from build123d import *

# Parameters (mm, degrees)
SKETCH_W      = 234
SKETCH_H      = 135
PAD_DEPTH     = 5
FILLET_R      = 3
FILLET001_R   = 3
FILLET002_R   = 3
FILLET003_R   = 3
SKETCH001_R   = 3
SKETCH001_R_2 = 5
POCKET_DEPTH  = 5.001


with BuildPart() as part:
    # Sketch → Pad (new body)
    with BuildSketch(Plane.XZ):
        Rectangle(SKETCH_W, SKETCH_H)
    extrude(amount=PAD_DEPTH)

    # Fillet
    fillet_edges = [part.edges().sort_by_distance(p)[0] for p in [
        (117, -2.5, 67.5),
    ]]
    fillet(fillet_edges, radius=FILLET_R)

    # Fillet001
    fillet001_edges = [part.edges().sort_by_distance(p)[0] for p in [
        (117, -2.5, -67.5),
    ]]
    fillet(fillet001_edges, radius=FILLET001_R)

    # Fillet002
    fillet002_edges = [part.edges().sort_by_distance(p)[0] for p in [
        (-117, -2.5, -67.5),
    ]]
    fillet(fillet002_edges, radius=FILLET002_R)

    # Fillet003
    fillet003_edges = [part.edges().sort_by_distance(p)[0] for p in [
        (-117, -2.5, 67.5),
    ]]
    fillet(fillet003_edges, radius=FILLET003_R)

    # Sketch001 (on Face10 of Fillet003) → Pocket (cut, through all)
    with BuildSketch(Plane.XZ.offset(5)):
        with Locations((-14.5, -47.5)):
            Circle(SKETCH001_R)
        with Locations((0, -47.5)):
            Circle(SKETCH001_R_2)
        with Locations((14.5, -47.5)):
            Circle(SKETCH001_R)
    extrude(amount=-POCKET_DEPTH, mode=Mode.SUBTRACT)


solid = part.part
Design review of the part built by this model. Coordinates are the model's own, in mm. Round coordinates to 2 decimals unless told otherwise and drop trailing zeros. Loops run counter-clockwise (first coordinate to the right, second up) from the corner with the lowest first, then second, coordinate; pieces in that order, holes last. Notation, with made-up numbers: (44, 10.25) - (74, 10.25) arc R28 ccw to (74, 48.25) - close; hole circle Ø11 at (46, 24.5). An arc over 180 degrees is marked (long way). One line per question, with ' | ' between items.
1. Clearance check with a flat-ended pin moving along its axis: P1, Ø13, axis at x = 0, z = -47.5, coming from the +Y side. State where the tip first meets the part, or that it passes through.
Results are:
P1: stops at y = 0
2. We need section A-A, the plane x = -14.5. State the section outline as (y, z) points, and give its area (3 significant figures).
Results are:
outline: (-5, -67.5) - (0, -67.5) - (0, -50.5) - (-5, -50.5) - close; (-5, -44.5) - (0, -44.5) - (0, 67.5) - (-5, 67.5) - close | area: 645 mm²
3. Draft analysis for pull direction X (two halves, no side actions). For faces 1 (the face through (-2, -2, 67.5)), 2 (the face through (117, -2, -1)), 3 (the face through (12.29, -2.54, -45.47)), 4 (the face through (-117, -2, -1)), state which applies: released by +X, released by -X, zero draft, split by the parting line, or undercut.
Results are:
face 1: zero draft | face 2: released by +X | face 3: undercut | face 4: released by -X
4. For L1, parallel to Z at x = 0, y = -3.4; L2, parallel to Z at x = 14.5, y = -2.3, list the stretches that pass through material, from the lowest coordinate up. Write a range as [from, to].
Results are:
L1: z = [-67.5, -52.5], [-42.5, 67.5] | L2: z = [-67.5, -50.5], [-44.5, 67.5]
